Part model, mm, in its own coordinate system. Coordinates: 2 decimals unless noted, no trailing zeros. Loops run counter-clockwise (first coordinate to the right, second up) from the corner with the lowest first, then second, coordinate; pieces in that order, holes last. Notation, with made-up numbers: M -18,36 L 21,36 A20 ccw 21,56 Z; hole C 32,12 d6. An arc over 180 degrees is marked long. Answer as CSV lines item,"result". Start each with the question number.
from build123d import *

# Parameters (mm, degrees)
BOSS_EXTRUDE1_DEPTH = 1.54


with BuildPart() as part:
    # Sketch1 → Boss-Extrude1 (new body)
    with BuildSketch(Plane.XY):
        with BuildLine():
            Line((7.939999995, -14.676928872), (7.939999995, 0))
            ThreePointArc((7.939999995, 0), (0, 7.939999995), (-7.939999995, 0))
            Line((-7.939999995, 0), (-7.939999995, -19.583493141))
            Line((-7.939999995, -19.583493141), (-5.090371955, -25.4))
            Line((-5.090371955, -25.4), (0.709510618, -25.4))
            Line((0.709510618, -25.4), (7.939999995, -14.676928872))
        make_face()
    extrude(amount=BOSS_EXTRUDE1_DEPTH)

    # Sketch3 → M6 Clearance Hole1 (revolve, cut)
    with BuildSketch(Plane.YZ):
        Polygon((0, 0), (0, 1.54), (3.3, 1.54), (3.3, 0.025), (3.325, 0), align=None)
    revolve(axis=Axis((0, 0, -6.35), (0, 0, 1)), mode=Mode.SUBTRACT)


solid = part.part
Q1. Slice it at C-C, the plane x = 5.5. Write the cut outline in (y, z), and give its area (3 significant figures).
Q2. Two-plate mould, pull along Y, no slides. Class faces 1 (the face through (0.17, 7.94, 0.76)), 2 (the face through (7.94, -7, 1)), 3 (the face through (4.274, -20.114, 0.759)), 4 (the face through (-2.23, -2.43, 0.77)): +Y half, -Y half, draft (parallel to the pull), parting line (faces both ways), or undercut.
Q3. Flat gauge pin, fed straight in: P1, Ø1, axis at x = 1, y = -2.5, coming from the +Z side. Where does the tip first touch, or does it go through?
Q4. Wall check: L1, parallel to Y at x = 0, z = 0.45; L2, parallel to Y at x = 3, z = 0.6; L3, parallel to X at y = -3, z = 0.4. Give the ranges that are in metal, low to high.
Q5. Slice it at B-B, the plane z = 0.3. Write the cut outline in (x, y), and give its area (3 significant figures).
Q6. Slice it at D-D, the plane y = 5.5. Write the cut outline in (x, z), and give its area (3 significant figures).
Q7. Slice it at A-A, the plane x = 0. Write the cut outline in (y, z) (3 decimals), and give its area (3 significant figures).
Solved:
1,outline,"M -18.3,0 L 5.73,0 L 5.73,1.54 L -18.3,1.54 Z"
1,area,"37.0 mm2"
2,face 1,"+Y half"
2,face 2,"draft"
2,face 3,"-Y half"
2,face 4,"undercut"
3,P1,"passes through"
4,L1,"y = -25.4 to -3.3, 3.3 to 7.94"
4,L2,"y = -22 to -1.37, 1.37 to 7.35"
4,L3,"x = -7.94 to -1.37, 1.37 to 7.94"
5,outline,"M -7.94,-19.58 L -5.09,-25.4 L 0.71,-25.4 L 7.94,-14.68 L 7.94,0 A7.94 ccw -7.94,0 Z; hole C 0,0 d6.6"
5,area,"421 mm2"
6,outline,"M -5.73,0 L 5.73,0 L 5.73,1.54 L -5.73,1.54 Z"
6,area,"17.6 mm2"
7,outline,"M -25.4,0 L -3.325,0 L -3.3,0.025 L -3.3,1.54 L -25.4,1.54 Z; M 3.3,0.025 L 3.325,0 L 7.94,0 L 7.94,1.54 L 3.3,1.54 Z"
7,area,"41.2 mm2"
